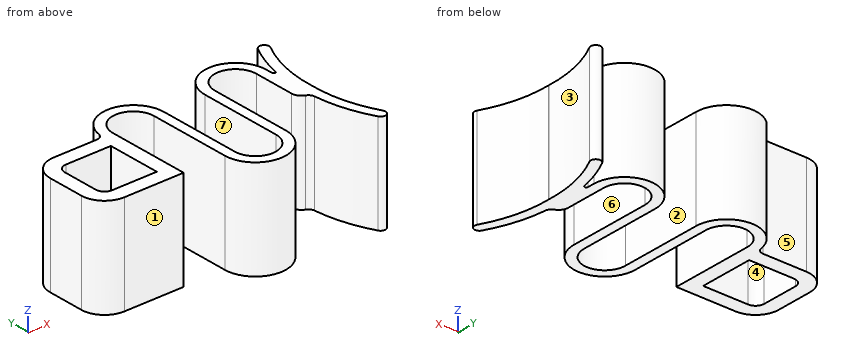
Autodesk Inventor part; units mm, degrees
ref_plane "YZ Plane" through (0, 0, 0) normal (1, 0, 0) x (0, 1, 0)
ref_plane "XZ Plane" through (0, 0, 0) normal (0, 1, 0) x (-1, 0, 0)
ref_plane "XY Plane" through (0, 0, 0) normal (0, 0, 1) x (1, 0, 0)
sketch "Boceto1" plane through (0, 0, 0) normal (0, 0, 1) x (1, 0, 0)
  line L0 (3, -11.4) -> (3, -5.5)
  line L1 (3, -5.5) -> (-2.2, -5.5)
  arc A0 (-5.5, -2.2) -> (-2.2, -5.5) centre (-2.2, -2.2) ccw
  line L2 (-5.5, -2.2) -> (-5.5, 2.2)
  arc A1 (-2.2, 5.5) -> (-5.5, 2.2) centre (-2.2, 2.2) ccw
  line L3 (-2.2, 5.5) -> (3, 5.5)
  line L4 (3, 5.5) -> (3, 11.4)
  line L5 (3, 3) -> (-2.2, 3)
  arc A2 (-2.2, 3) -> (-3, 2.2) centre (-2.2, 2.2) ccw
  line L6 (-3, 2.2) -> (-3, -2.2)
  arc A3 (-3, -2.2) -> (-2.2, -3) centre (-2.2, -2.2) ccw
  line L7 (-2.2, -3) -> (3, -3)
  line L8 (3, -3) -> (3, 3)
  line L9 (-2.2, 3.25) -> (3.25, 3.25)
  line L10 (3.25, 3.25) -> (3.25, -3.25)
  line L11 (3.25, -3.25) -> (-2.2, -3.25)
  arc A4 (-3.25, -2.2) -> (-2.2, -3.25) centre (-2.2, -2.2) ccw
  line L12 (-3.25, -2.2) -> (-3.25, 2.2)
  arc A5 (-2.2, 3.25) -> (-3.25, 2.2) centre (-2.2, 2.2) ccw
  line L13 (-2.2, 5) -> (5, 5)
  line L14 (5, 5) -> (5, -5)
  line L15 (5, -5) -> (-2.2, -5)
  arc A6 (-5, -2.2) -> (-2.2, -5) centre (-2.2, -2.2) ccw
  line L16 (-5, -2.2) -> (-5, 2.2)
  arc A7 (-2.2, 5) -> (-5, 2.2) centre (-2.2, 2.2) ccw
  line L17 (5, 5) -> (7.5, 5)
  line L18 (10, 5) -> (11.2, 5)
  line L19 (11.2, 5) -> (11.2, -5)
  line L20 (11.2, -5) -> (10, -5)
  line L21 (10, -5) -> (10, 5)
  line L22 (11.2, -5) -> (13.7, -5)
  line L23 (16.2, -5) -> (17.4, -5)
  line L24 (17.4, -5) -> (17.4, 5)
  line L25 (17.4, 5) -> (16.2, 5)
  line L26 (16.2, 5) -> (16.2, -5)
  line L27 (17.4, 5) -> (19.9, 5)
  line L28 (22.4, 5) -> (23.6, 5)
  line L29 (23.6, 5) -> (23.6, 0)
  line L30 (23.6, 0) -> (22.4, 0)
  line L31 (22.4, 0) -> (22.4, 5)
  arc A8 (11.2, 5) -> (3.8, 5) centre (7.5, 5) ccw
  arc A9 (10, 5) -> (5, 5) centre (7.5, 5) ccw
  arc A10 (10, -5) -> (17.4, -5) centre (13.7, -5) ccw
  arc A11 (11.2, -5) -> (16.2, -5) centre (13.7, -5) ccw
  arc A12 (22.4, 5) -> (17.4, 5) centre (19.9, 5) ccw
  arc A13 (23.6, 5) -> (16.2, 5) centre (19.9, 5) ccw
  arc A14 (25.6, 8.5) -> (23.6, 0) centre (40.821, 0.4333) ccw
  circle A15 centre (23.6, 0) radius 1.2
  arc A16 (26.6603, 7.9381) -> (24.7996, 0.0302) centre (40.821, 0.4333) ccw
  line L32 (25.6, 8.5) -> (25.9736, 8.302)
  arc A17 (26.6603, 7.9381) -> (25.6, 8.5) centre (26.1301, 8.219) ccw
  arc A18 (23.6, 0) -> (25.6, -8.5) centre (40.821, -0.4333) ccw
  arc A19 (24.7996, -0.0302) -> (26.6603, -7.9381) centre (40.821, -0.4333) ccw
  line L33 (25.9736, -8.302) -> (26.6603, -7.9381)
  arc A20 (25.6, -8.5) -> (26.6603, -7.9381) centre (26.1301, -8.219) ccw
  point P0 (0, 0)
  point P1 (5, -5)
  point P2 (4.2, -5)
  point P3 (23, 0)
  point P4 (23.6, 1.2)
  point P5 (23.6116, -1.1999)
  point P6 (24.7996, 0.0302)
  point P7 (23.6116, 1.1999)
  dimension "d1" = 0.25
  dimension "d2" = 2
  dimension "d31" = 2.5
  dimension "d33" = 10
  dimension "d34" = 2.5
  dimension "d35" = 1.2
  dimension "d36" = 10
  dimension "d37" = 2.5
  dimension "d41" = 1.2
extrude "Extrusión1" add sketch "Boceto1" along normal blind 12 contours L13 L14 L15 A6 L16 A7 | A8 L18 A9 L13 | L19 L20 L21 L18 | A11 L23 A10 L20 | L26 L25 L24 L23 | A13 L28 A12 L25 | L29 A15 L31 L28 | A15 A14 L29 | L29 A14 L30 A15 | L30 A18 A15 | A14 A15 A18 L29 | L29 A14 | A14 A17 A16 A15 | A15 A19 A20 A18
fillet "Empalme1" radius 0.8 2 edges at (3.8, 5, 6) (23.6116, -1.1999, 6)
fillet "Empalme1" radius 0.2 2 edges at (23.6, 1.2, 6) (23.6116, 1.1999, 6)
properties part number "_3DPrint"
CAD build for the part. Positions are in the model's coordinates, mm. Face numbers are marked on the shaded views. A direction names the side the tool comes from. Coordinates: 2 decimals unless noted, no trailing zeros. Write each loop counter-clockwise with the first axis right and the second up, starting at its lowest first coordinate (ties: lowest second). Pieces come first, ordered by that corner, then holes. Notation, with made-up numbers: M 35,-13.75 L 74,-13.75 A29 cw 74,25.25 Z; hole C 42,54.25 d11. An arc over 180 degrees is marked long. Answer as a JSON object with one key per item and string values. Group by question number.
1) Saw through at C-C (x = 19.9). Write the cut outline in (y, z).
2) Saw through at B-B (y = -5.5). Write the cut outline in (x, z), plus the area to 3 significant figures.
3) Tool access for the marked faces 4, 5, 6 and 7: list every direction of +Z, -Z, +X, -X, +Y, -Y with a clear straight run to the whole face (end or side of a thin tool).
4) Saw through at A-A (x = 2.5). Write the cut outline in (y, z).
5) Pin check, flat tips, straight feed: pin 1 Ø1.5 at (x, z) = (7.5, 8) entering from +Y; pin 2 Ø2 at (x, y) = (2, 2) entering from -Z; pin 3 Ø2.5 at (x, z) = (-1, 6.5) entering from +Y; pin 4 Ø1.6 at (x, z) = (1.5, 9) entering from -Y. Stop position of each tip, or through.
6) Mould opens along X. For the marked faces 1, 2 and 3 say: +X half, -X half, draft (parallel to the pull), parting line (faces both ways), or undercut.
7) Saw through at D-D (x = 6.5). Write the cut outline in (y, z), plus the area to 3 significant figures.
8) Wall check: line 1 (Y direction, x = -2, z = 7.5); line 2 (X direction, y = 5.5, z = 2.25); line 3 (X direction, y = -4, z = 6). Give the ranges that are in metal, low to high. Write a range as from..to.
Values follow:
{
 "1": {"outline": "M 7.5,0 L 8.7,0 L 8.7,12 L 7.5,12 Z"},
 "2": {"outline": "M 10.03,0 L 11.25,0 L 11.25,12 L 10.03,12 Z; M 16.15,0 L 17.37,0 L 17.37,12 L 16.15,12 Z; M 24.36,0 L 25.62,0 L 25.62,12 L 24.36,12 Z", "area": "44.3 mm2"},
 "3": {"face 4": "+Z, -Z", "face 5": "+Z, -Z, -X, +Y", "face 6": "+Z, -Z, -Y", "face 7": "+Z, -Z, +Y"},
 "4": {"outline": "M -5,0 L -3.25,0 L -3.25,12 L -5,12 Z; M 3.25,0 L 5,0 L 5,12 L 3.25,12 Z"},
 "5": {"pin 1": "stops at y = 8.7", "pin 2": "passes through", "pin 3": "stops at y = 5", "pin 4": "stops at y = -5"},
 "6": {"face 1": "draft", "face 2": "undercut", "face 3": "+X half"},
 "7": {"outline": "M 7.29,0 L 8.56,0 L 8.56,12 L 7.29,12 Z", "area": "15.3 mm2"},
 "8": {"line 1": "y = -5..-3.25, 3.25..5", "line 2": "x = 3.81..5.05, 9.95..11.17, 16.23..17.45, 22.35..23.57, 24.36..25.62", "line 3": "x = -4.34..5, 10..11.2, 16.2..17.4, 23.97..25.2"}
}
